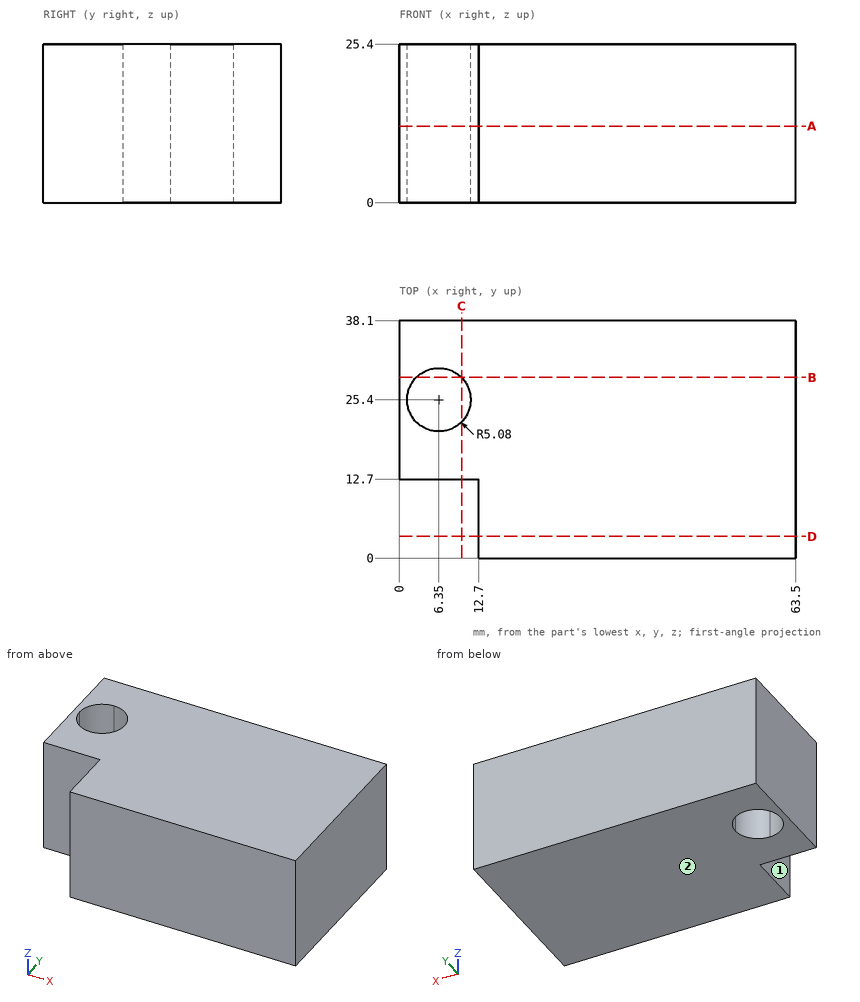
Geometry check sheet. Reference: drawing and pictorial views, mm from the part's lowest x, y, z. A direction names the side the tool comes from. Round coordinates to 2 decimals unless told otherwise and drop trailing zeros. Loops run counter-clockwise (first coordinate to the right, second up) from the corner with the lowest first, then second, coordinate; pieces in that order, holes last. Notation, with made-up numbers: M -27.5,-27.75 L -19.5,-27.75 A26 cw -19.5,4.25 Z; hole C 75,12 d8. An arc over 180 degrees is marked long. Return JSON: item names as keys, results as strings. Group by question number.
(1) Go/stop test with flat-tipped pins: pin 1 (8 mm diameter, centred on y = 6.5, z = 21, fed in from -X); pin 2 (14 mm diameter, centred on x = 4.5, z = 16.5, fed in from -Y); pin 3 (10 mm diameter, centred on x = 29, y = 17.5, fed in from -Z); pin 4 (6 mm diameter, centred on x = 7, y = 4, fed in from -Z). Record where each tip stops, or that it passes through.
(2) Section check C-C, the plane x = 10. Enter the section's corners in (y, z), and give its area (3 significant figures).
(3) Set-up check for the marked faces 1 and 2: record each of +Z, -Z, +X, -X, +Y, -Y from which the full face is reachable in a straight line by a thin tool's end or side.
(4) Scan lines: line 1 along X through (y, z) = (9, 23.5); line 2 along X through (y, z) = (21, 24); line 3 along X through (y, z) = (27, 12.5). Record each from-to range of solid material in increasing order. Write a range as [from, to].
(5) Section check A-A, the plane z = 12.25. Enter the section's corners in (x, y).
(6) Section check D-D, the plane y = 3.5. Enter the section's corners in (x, z).
(7) Section check B-B, the plane y = 29. Enter the section's corners in (x, z).
Data:
{
 "1": {"pin 1": "x = 12.7", "pin 2": "y = 12.7", "pin 3": "z = 0", "pin 4": "through"},
 "2": {"outline": "M 12.7,0 L 21.87,0 L 21.87,25.4 L 12.7,25.4 Z; M 28.93,0 L 38.1,0 L 38.1,25.4 L 28.93,25.4 Z", "area": "466 mm²"},
 "3": {"face 1": "+Z, -Z, -X, -Y", "face 2": "-Z, +X, -X, +Y, -Y"},
 "4": {"line 1": "[12.7, 63.5]", "line 2": "[0, 3.81], [8.89, 63.5]", "line 3": "[0, 1.53], [11.17, 63.5]"},
 "5": {"outline": "M 0,12.7 L 12.7,12.7 L 12.7,0 L 63.5,0 L 63.5,38.1 L 0,38.1 Z; hole M 1.27,25.4 A5.08 ccw 6.35,20.32 A5.08 ccw 11.43,25.4 A5.08 ccw 6.35,30.48 A5.08 ccw Z"},
 "6": {"outline": "M 12.7,0 L 63.5,0 L 63.5,25.4 L 12.7,25.4 Z"},
 "7": {"outline": "M 0,0 L 2.77,0 L 2.77,25.4 L 0,25.4 Z; M 9.93,0 L 63.5,0 L 63.5,25.4 L 9.93,25.4 Z"}
}
